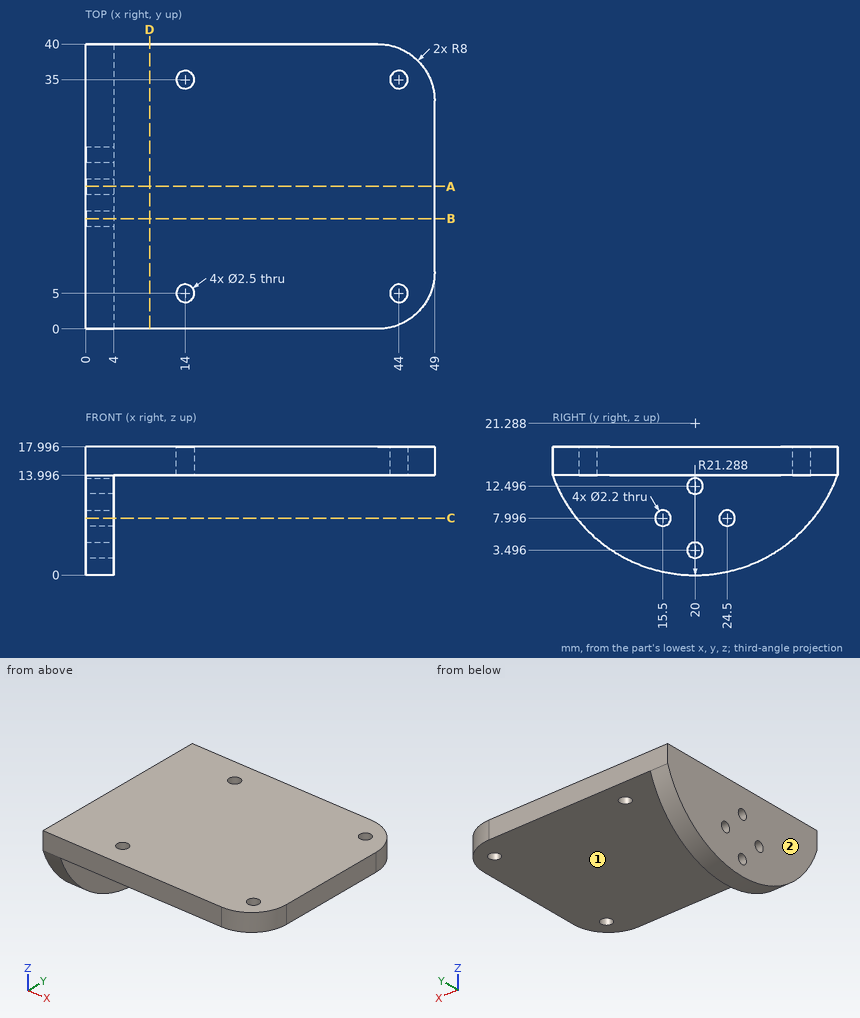
Part print with two shaded views. Sizes in mm from the minimum x, y, z corner. A direction names the side the tool comes from. Coordinates: 2 decimals unless noted, no trailing zeros. Write each loop counter-clockwise with the first axis right and the second up, starting at its lowest first coordinate (ties: lowest second). Pieces come first, ordered by that corner, then holes.
(1) Pin check, flat tips, straight feed: pin 1 Ø3.5 at (y, z) = (24.5, 8) entering from +X; pin 2 Ø3 at (x, y) = (14, 35) entering from -Z. Stop position of each tip, or through.
(2) Cut at A-A on y = 20. List the corners of the cut face in (x, z).
(3) 3-axis set-ups, long thin cutter, end or side, ignore diameter. For the marked faces 1 and 2: which of +Z, -Z, +X, -X, +Y, -Y reach the whole face in a straight line?
(4) Cut at C-C on z = 8. List the corners of the cut face in (x, y).
(5) Drill centre lines: line 1 (Y direction, x = 14, z = 14.8); line 2 (Z direction, x = 24.5, y = 23); line 3 (X direction, y = 18, z = 10.25). Where is each one in solid material? Low to high.
(6) Cut at B-B on y = 15.5. List the corners of the cut face in (x, z).
(7) Cut at D-D on x = 9. List the corners of the cut face in (y, z).
Working result:
1. pin 1: stops at x = 4
1. pin 2: stops at z = 14
2. outline: (0, 0) - (4, 0) - (4, 2.4) - (0, 2.4) - close; (0, 4.6) - (4, 4.6) - (4, 11.4) - (0, 11.4) - close; (0, 13.6) - (4, 13.6) - (4, 14) - (49, 14) - (49, 18) - (0, 18) - close
3. face 1: -Z, +X, +Y, -Y
3. face 2: +Z, -Z, -X, +Y, -Y
4. outline: (0, 3.37) - (4, 3.37) - (4, 14.4) - (0, 14.4) - close; (0, 16.6) - (4, 16.6) - (4, 23.4) - (0, 23.4) - close; (0, 25.6) - (4, 25.6) - (4, 36.63) - (0, 36.63) - close
5. line 1: y = 0 to 3.75, 6.25 to 33.75, 36.25 to 40
5. line 2: z = 14 to 18
5. line 3: x = 0 to 4
6. outline: (0, 0.48) - (4, 0.48) - (4, 6.9) - (0, 6.9) - close; (0, 9.1) - (4, 9.1) - (4, 14) - (49, 14) - (49, 18) - (0, 18) - close
7. outline: (0, 14) - (40, 14) - (40, 18) - (0, 18) - close
